Part model, mm, in its own coordinate system. A direction names the side the tool comes from. Round coordinates to 2 decimals unless told otherwise and drop trailing zeros. Loops run counter-clockwise (first coordinate to the right, second up) from the corner with the lowest first, then second, coordinate; pieces in that order, holes last.
(1) Cut at A-A on z = 4.5. List the corners of the cut face in (x, y) (3 decimals).
(2) Tool access for faces 4 (the face through (8, 27, 15)), 5 (the face through (53, -55, 7)), 6 (the face through (45.53, 15, 7)), 7 (the face through (-35, -55, 7)), 8 (the face through (-27.86, 15, 7)): list every direction of +Z, -Z, +X, -X, +Y, -Y with a clear straight run to the whole face (end or side of a thin tool).
(3) Mould opens along X. For faces 1 (the face through (45.53, -65, 7)), 2 (the face through (-4.152, 75.572, 7.395)), 3 (the face through (-35, 5, 7)) say: +X half, -X half, draft (parallel to the pull), parting line (faces both ways), or undercut.
(4) Flat gauge pins, fed straight in: pin 1 (7.5 mm diameter, centred on x = 53.5, z = 7.5, fed in from -Y); pin 2 (8 mm diameter, centred on y = 78, z = 3, fed in from +X); pin 3 (7.5 mm diameter, centred on y = 17, z = 4, fed in from -X); pin 4 (5 mm diameter, centred on x = 22.5, z = 7, fed in from +Y). Where does each tip first touch, or does it go through?
(5) Cut at B-B on y = 100.5. List the corners of the cut face in (x, z).
(6) Probe probe 1 along Y at (x, z) = (-34.5, 5); probe 2 along X at (y, z) = (23, 7.75); probe 3 along Y at (x, z) = (1.5, 13.25). List the from-to ranges inside material, lowest first.
(7) Cut at C-C on x = -21. List the corners of the cut face in (y, z).
from build123d import *

# Parameters (mm, degrees)
ESQUISSE1_R        = 13
BOSS_EXTRU_1_DEPTH = 15


with BuildPart() as part:
    # Esquisse1 → Boss.-Extru.1 (new body)
    with BuildSketch(Plane.XY):
        with BuildLine():
            Line((-27.86, -55), (-27.86, -75))
            Line((-27.86, -75), (45.53, -75))
            Line((45.53, -75), (45.53, -55))
            Line((45.53, -55), (60.53, -55))
            Line((60.53, -55), (60.53, 5))
            Line((60.53, 5), (45.53, 5))
            Line((45.53, 5), (45.53, 25))
            Line((45.53, 25), (60.53, 25))
            Line((60.53, 25), (60.53, 75))
            ThreePointArc((60.53, 75), (8.835, 126.695), (-42.86, 75))
            Line((-42.86, 75), (-42.86, 25))
            Line((-42.86, 25), (-27.86, 25))
            Line((-27.86, 25), (-27.86, 5))
            Line((-27.86, 5), (-42.86, 5))
            Line((-42.86, 5), (-42.86, -55))
            Line((-42.86, -55), (-27.86, -55))
        make_face()
        with Locations((8.835, 75)):
            Circle(ESQUISSE1_R, mode=Mode.SUBTRACT)
    extrude(amount=BOSS_EXTRU_1_DEPTH)


solid = part.part
Final values:
1. outline: (-42.86, -55) - (-27.86, -55) - (-27.86, -75) - (45.53, -75) - (45.53, -55) - (60.53, -55) - (60.53, 5) - (45.53, 5) - (45.53, 25) - (60.53, 25) - (60.53, 75) arc R51.695 ccw to (-42.86, 75) - (-42.86, 25) - (-27.86, 25) - (-27.86, 5) - (-42.86, 5) - close; hole circle Ø26 at (8.835, 75)
2. face 4: +Z, +X, -X, +Y, -Y
2. face 5: +Z, -Z, +X, -Y
2. face 6: +Z, -Z, +X
2. face 7: +Z, -Z, -X, -Y
2. face 8: +Z, -Z, -X
3. face 1: +X half
3. face 2: undercut
3. face 3: draft
4. pin 1: stops at y = -55
4. pin 2: stops at x = 60.53
4. pin 3: stops at x = -27.86
4. pin 4: stops at y = 125.47
5. outline: (-36.13, 0) - (53.8, 0) - (53.8, 15) - (-36.13, 15) - close
6. probe 1: y = -55 to 5, 25 to 103.19
6. probe 2: x = -27.86 to 45.53
6. probe 3: y = -75 to 64.27, 85.73 to 126.17
7. outline: (-75, 0) - (117.22, 0) - (117.22, 15) - (-75, 15) - close
